Print and shaded views of the part. All mm, measured from the part's lowest x, y and z. Give positions to 0.01 mm unless a question says otherwise; leave off trailing zeros. Loops run counter-clockwise (first coordinate to the right, second up) from the corner with the lowest first, then second, coordinate; pieces in that order, holes last. Notation, with made-up numbers: (-17.75, 83.5) - (4.25, 83.5) arc R22 ccw to (4.25, 93.5) - close; hole circle Ø4 at (41, 48). An arc over 180 degrees is marked (long way). Return JSON: item names as keys, results as strings.
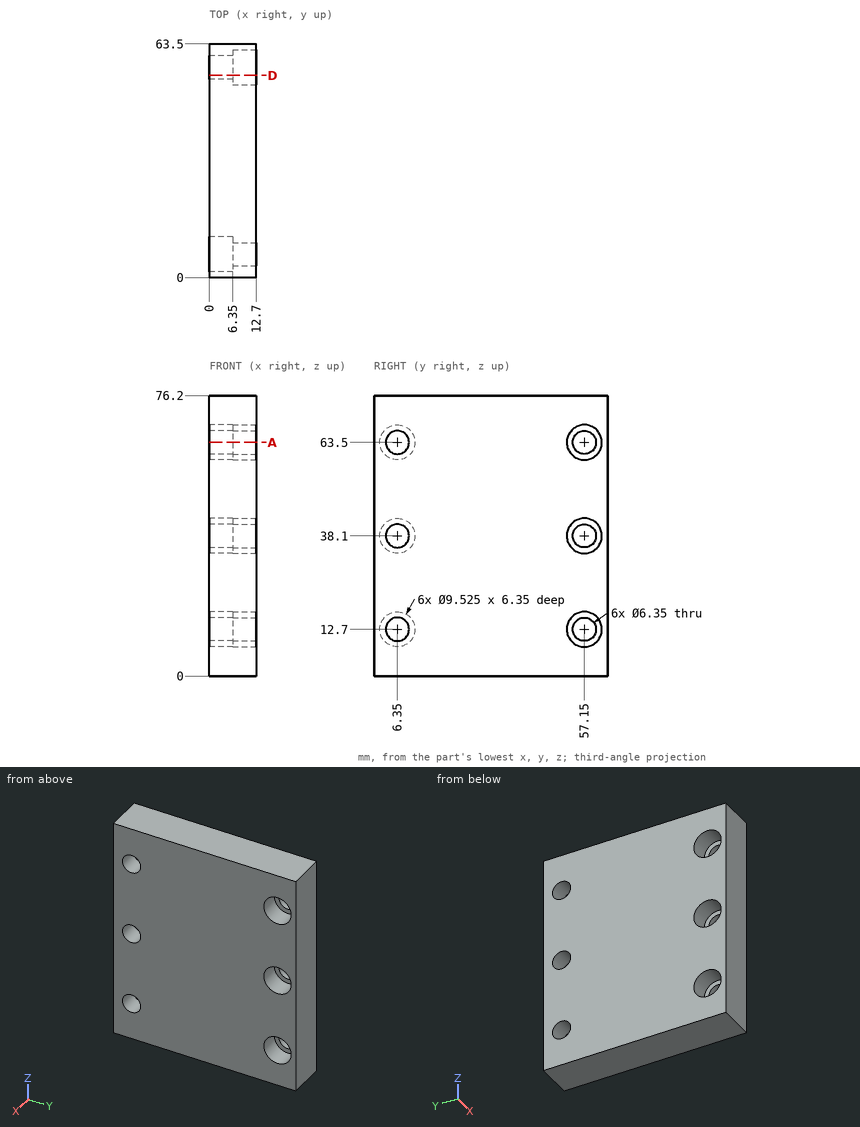
1. Cut at A-A, the plane z = 63.5. Give the number of separate pieces and of enclosed holes in the cut face, plus the area to 3 significant figures.
Values follow:
{"separate pieces": "3", "enclosed holes": "0", "area": "605 mm²"}
2. Drill centre lines: probe 1 along Y at (x, z) = (3.75, 63.5) (1 decimal); probe 2 along Z at (x, y) = (5.25, 55); probe 3 along Z at (x, y) = (7.75, 6). Where is each one in solid material? Low to high.
Values follow:
{"probe 1": "y = 0 to 1.6, 11.1 to 54, 60.3 to 63.5", "probe 2": "z = 0 to 10.36, 15.04 to 35.76, 40.44 to 61.16, 65.84 to 76.2", "probe 3": "z = 0 to 9.54, 15.86 to 34.94, 41.26 to 60.34, 66.66 to 76.2"}
3. Drop flat-ended pins along their axis: P1, Ø5, axis at y = 6.35, z = 38.1, coming from the -X side; P2, Ø3, axis at y = 8, z = 15, coming from the -X side; P3, Ø5, axis at y = 57.5, z = 11.5, coming from the +X side. Give the stop position or say it passes through.
Values follow:
{"P1": "passes through", "P2": "stops at x = 6.35", "P3": "stops at x = 6.35"}
4. Cut at D-D, the plane y = 55. Write the cut outline in (x, z).
Values follow:
{"outline": "(0, 0) - (12.7, 0) - (12.7, 8.45) - (6.35, 8.45) - (6.35, 10.36) - (0, 10.36) - close; (0, 15.04) - (6.35, 15.04) - (6.35, 16.95) - (12.7, 16.95) - (12.7, 33.85) - (6.35, 33.85) - (6.35, 35.76) - (0, 35.76) - close; (0, 40.44) - (6.35, 40.44) - (6.35, 42.35) - (12.7, 42.35) - (12.7, 59.25) - (6.35, 59.25) - (6.35, 61.16) - (0, 61.16) - close; (0, 65.84) - (6.35, 65.84) - (6.35, 67.75) - (12.7, 67.75) - (12.7, 76.2) - (0, 76.2) - close"}
